```python
from build123d import *

# Parameters (mm, degrees)
SKETCH2_R           = 3.175
BOSS_EXTRUDE1_DEPTH = 5.08


with BuildPart() as part:
    # Sketch2 → Boss-Extrude1 (new body)
    with BuildSketch(Plane.XY):
        with BuildLine():
            Line((-95.458507722, -102.59724), (-102.247977436, -99.137832392))
            Line((-102.247977436, -99.137832392), (-105.707385044, -105.927302106))
            Line((-105.707385044, -105.927302106), (-98.91791533, -109.386709714))
            Line((-98.91791533, -109.386709714), (-111.025841958, -133.149853715))
            ThreePointArc((-111.025841958, -133.149853715), (-95.109842937, -182.134261878), (-46.125434774, -166.218262858))
            Line((-46.125434774, -166.218262858), (0, -75.692))
            Line((0, -75.692), (0, -7.62))
            Line((0, -7.62), (7.62, -7.62))
            Line((7.62, -7.62), (7.62, 0))
            Line((7.62, 0), (0, 0))
            Line((0, 0), (-75.278630008, 0))
            Line((-75.278630008, 0), (-75.278630008, -62.992))
            Line((-75.278630008, -62.992), (-95.458507722, -102.59724))
        make_face()
        with Locations((3.81, -3.81)):
            Circle(SKETCH2_R, mode=Mode.SUBTRACT)
        with Locations((-100.582946383, -104.262271053)):
            Circle(SKETCH2_R, mode=Mode.SUBTRACT)
    extrude(amount=BOSS_EXTRUDE1_DEPTH)


solid = part.part
```
Geometry check sheet. Reference: the model listing, model coordinates, mm. A direction names the side the tool comes from. Round coordinates to 2 decimals unless told otherwise and drop trailing zeros. Write each loop counter-clockwise with the first axis right and the second up, starting at its lowest first coordinate (ties: lowest second). Pieces come first, ordered by that corner, then holes. Notation, with made-up numbers: (60, 46) - (116, 46) arc R22 cw to (116, 83) - close; hole circle Ø2 at (-31, -2). An arc over 180 degrees is marked (long way). Write each question's results on one line, items separated by ' | '.
(1) Thickness scan on probe 1 along Y at (x, z) = (3.81, 1.35) (3 decimals); probe 2 along X at (y, z) = (-57.5, 1.85); probe 3 along X at (y, z) = (-95.5, 2.75). Record the ranges inside material, lowest first. Write a range as from..to.
Computed:
probe 1: y = -7.62..-6.985, -0.635..0 | probe 2: x = -75.28..0 | probe 3: x = -91.84..-10.09
(2) Sectioned sample at B-B, the plane y = -3.81. Enter the section's corners in (x, z) (3 decimals), plus the area to 3 significant figures.
Computed:
outline: (-75.279, 0) - (0.635, 0) - (0.635, 5.08) - (-75.279, 5.08) - close; (6.985, 0) - (7.62, 0) - (7.62, 5.08) - (6.985, 5.08) - close | area: 389 mm^2
(3) Draft check along X on faces 5 (the face through (-95.819, -181.763, 2.504)), 6 (the face through (4, -7.62, 3)), 7 (the face through (-102.923, -102.116, 2.504)), 8 (the face through (-75.279, -31, 3)). Enter one of: pulls with the +X half, pulls with the -X half, needs draft (parallel to the pull), parting line crosses it, or undercut.
Computed:
face 5: parting line crosses it | face 6: needs draft | face 7: undercut | face 8: pulls with the -X half
(4) Sectioned sample at C-C, the plane z = 2.95. Count the separate pieces of the cut face and the enclosed holes in it, plus the area to 3 significant figures.
Computed:
separate pieces: 1 | enclosed holes: 2 | area: 13,900 mm^2
(5) Set-up check for faces 1 (the face through (0, -42, 3)), 2 (the face through (-33, 0, 3)), 3 (the face through (-98.81, -100.89, 2.5)), 4 (the face through (-102.36, -107.633, 2.504)): record each of +Z, -Z, +X, -X, +Y, -Y from which the full face is reachable in a straight line by a thin tool's end or side.
Computed:
face 1: +Z, -Z, +X, -Y | face 2: +Z, -Z, +X, -X, +Y | face 3: +Z, -Z, +Y | face 4: +Z, -Z, -X
(6) Sectioned sample at A-A, the plane x = 3.81. Enter the section's corners in (y, z) (3 decimals), plus the area to 3 significant figures.
Computed:
outline: (-7.62, 0) - (-6.985, 0) - (-6.985, 5.08) - (-7.62, 5.08) - close; (-0.635, 0) - (0, 0) - (0, 5.08) - (-0.635, 5.08) - close | area: 6.45 mm^2
(7) Depth check by flat-ended pin: pin 1 Ø2 at (x, y) = (-34.5, -93.5) entering from -Z; pin 2 Ø1.5 at (y, z) = (-49, 1.5) entering from +X; pin 3 Ø5 at (x, y) = (3.81, -3.81) entering from +Z; pin 4 Ø1.5 at (y, z) = (-95.5, 2) entering from +X. Enter the tip coordinate at first touch or a pass-through.
Computed:
pin 1: stops at z = 0 | pin 2: stops at x = 0 | pin 3: passes through | pin 4: stops at x = -9.71
(8) Sectioned sample at D-D, the plane y = -47. Enter the section's corners in (x, z).
Computed:
outline: (-75.28, 0) - (0, 0) - (0, 5.08) - (-75.28, 5.08) - close
